```python
from build123d import *

# Parameters (mm, degrees)
F5_R = 10


with BuildPart() as f6:
    # F6: sweep along a path in F0, F4, F2
    with BuildLine(Plane.XZ) as f6_path:
        Line((0, 0), (10, 0))
        ThreePointArc((10, 0), (24.1421356237, -5.8578643763), (30, -20))
        Line((30, -20), (30, -602.5))
    with BuildLine(Plane.YZ.offset(30)) as f6_path_2:
        ThreePointArc((0, -602.5), (5.8578643763, -616.6421356237), (20, -622.5))
    with BuildLine(Plane.XY.offset(-622.5)) as f6_path_3:
        Line((30, 20), (30, 190.785))
        ThreePointArc((30, 190.785), (35.8578643763, 204.9271356237), (50, 210.785))
        Line((50, 210.785), (159.583, 210.785))
    # F5 (on Right) → F6 (sweep)
    with BuildSketch(Plane.YZ):
        Circle(F5_R)
    sweep(path=f6_path.line + f6_path_2.line + f6_path_3.line)


solid = f6.part
```
Design review of the part built by this model. Coordinates are the model's own, in mm. A direction names the side the tool comes from. Coordinates: 2 decimals unless noted, no trailing zeros. Order: outer loops, then holes, each group sorted by start corner. A loop starts at its lowest first (then second) coordinate and runs counter-clockwise, first axis right, second up. Notation, with made-up numbers: (75.5, 82.25) -> (92.5, 82.25) arc R12 cw to (92.5, 104.25) -> close; hole circle Ø5 at (65, 32.5). An arc over 180 degrees is marked (long way). One line per item, written item: value. Start each with the question number.
Q1. Tool access review of faces 4 (the cylindrical face through (26.17, 106.588, -613.263)), 5 (the flat face through (159.583, 211, -623)), 6 (the cylindrical face through (105.559, 207.781, -612.962)): name each direction out of +Z, -Z, +X, -X, +Y, -Y from which nothing blocks a thin tool from reaching the whole face with its end or side.
Q2. Insertion check: pin 1 Ø1 at (x, y) = (23, 175.5) entering from +Z; pin 2 Ø6 at (x, y) = (29.5, 76.5) entering from -Z; pin 3 Ø4 at (x, y) = (34, 106) entering from +Z. Each pin has a flat end and moves straight along its axis. Give the tip position at first contact, or say it passes through.
Q3. For probe 1 along Y at (x, z) = (29.5, -593.5); probe 2 along Z at (x, y) = (32, 127); probe 3 along Z at (x, y) = (38, 152), list the stretches that pass through material, from the lowest coordinate up.
Q4. Take a section at A-A, the plane y = 132. State the section outline as (x, z) points, then the cut area to 3 significant figures.
Q5. Take a section at B-B, the plane z = -463.5. State the section outline as (x, y) points, then the cut area to 3 significant figures.
Q6. Mouldability with a two-part tool opening along Z and no side actions: class faces 1 (the cylindrical face through (5.07, -2.17, -9.76)), 2 (the cylindrical face through (20.24, -2.17, -315.33)), 3 (the flat face through (0, 0, 0)) as pulls with the +Z half, pulls with the -Z half, needs draft (parallel to the pull), parting line crosses it, or undercut.
Values follow:
1. face 4: none
1. face 5: +Z, -Z, +X, +Y, -Y
1. face 6: +X
2. pin 1: stops at z = -614.9
2. pin 2: stops at z = -632.5
2. pin 3: stops at z = -612.7
3. probe 1: y = -9.99 to 9.99
3. probe 2: z = -632.3 to -612.7
3. probe 3: z = -628.5 to -616.5
4. outline: circle Ø20 at (30, -622.5)
4. area: 314 mm2
5. outline: circle Ø20 at (30, 0)
5. area: 314 mm2
6. face 1: parting line crosses it
6. face 2: undercut
6. face 3: needs draft
